Verification items for the finished model (mm, model axes). A direction names the side the tool comes from. Round coordinates to 2 decimals unless told otherwise and drop trailing zeros. Write each loop counter-clockwise with the first axis right and the second up, starting at its lowest first coordinate (ties: lowest second). Pieces come first, ordered by that corner, then holes. Notation, with made-up numbers: M -26,13 L 10,13 A18 cw 10,44 Z; hole C -18,57 d3. An arc over 180 degrees is marked long. One line per question, with ' | ' between items. Start each with the question number.
Q1. Gauge pin test, flat ends, axial feed: pin 1 (1.5 mm diameter, centred on x = -3.5, y = 11.5, fed in from -Z); pin 2 (3.5 mm diameter, centred on x = 14, y = -61.5, fed in from +Z). Record the tip position at first contact, or that the pin passes through.
Q2. Cross-section at C-C (z = 12.5). State how many separate pieces and enclosed holes the cut face has, then the cut area to 3 significant figures.
Q3. Tool access check on faces 1 (the face through (14, -61, 10)), 2 (the face through (25, -1, 7)). Record the directions out of +Z, -Z, +X, -X, +Y, -Y that give a thin tool (end or side, any length) a straight path to the whole face; none if there is none.
Q4. Cross-section at D-D (y = 21.18). Record the boundary of the cut face in (x, z).
Q5. Thickness scan on line 1 along Y through (x, z) = (-16.5, 12.85); line 2 along Y through (x, z) = (-10, 5.25); line 3 along X through (y, z) = (-14, 7.5). Record the ranges inside material, lowest first. Write a range as from..to.
Q6. Cross-section at B-B (y = 59.5). Record the boundary of the cut face in (x, z).
Q7. Release check for a two-part mould opening along Y. For faces 3 (the face through (15.784, -54.047, 12.535)), 4 (the face through (23, 67, 8)), 5 (the face through (0, -68, 7)) record: released by +Y, released by -Y, zero draft, split by the parting line, or undercut.
Q8. Cross-section at A-A (x = 16.5). Record the boundary of the cut face in (y, z).
from build123d import *

# Parameters (mm, degrees)
SKETCH_W        = 50
SKETCH_H        = 136
PAD_DEPTH       = 15
SKETCH001_R     = 2.75
POCKET_DEPTH    = 15.001
SKETCH002_R     = 5.5
POCKET001_DEPTH = 5
SKETCH003_R     = 2
POCKET002_DEPTH = 15.001
FILLET_R        = 5


with BuildPart() as part:
    # Sketch → Pad (new body)
    with BuildSketch(Plane.XY):
        Rectangle(SKETCH_W, SKETCH_H)
    extrude(amount=PAD_DEPTH)

    # Sketch001 (on Face6 of Pad) → Pocket (cut, through all)
    with BuildSketch(Plane.XY.offset(15)):
        with Locations((-16.5, 59.5)):
            Circle(SKETCH001_R)
        with Locations((16.5, 59.5)):
            Circle(SKETCH001_R)
        with Locations((16.5, -59.5)):
            Circle(SKETCH001_R)
        with Locations((-16.5, -59.5)):
            Circle(SKETCH001_R)
    extrude(amount=-POCKET_DEPTH, mode=Mode.SUBTRACT)

    # Sketch002 (on Face5 of Pocket) → Pocket001 (cut)
    with BuildSketch(Plane.XY.offset(15)):
        with Locations((-16.5, -59.5)):
            Circle(SKETCH002_R)
        with Locations((16.5, -59.5)):
            Circle(SKETCH002_R)
        with Locations((16.5, 59.5)):
            Circle(SKETCH002_R)
        with Locations((-16.5, 59.5)):
            Circle(SKETCH002_R)
    extrude(amount=-POCKET001_DEPTH, mode=Mode.SUBTRACT)

    # Sketch003 (on Face5 of Pocket001) → Pocket002 (cut, through all)
    with BuildSketch(Plane.XY.offset(15)):
        with Locations((10, 21.18)):
            Circle(SKETCH003_R)
        with Locations((-10, 21.18)):
            Circle(SKETCH003_R)
        with Locations((10, -14.82)):
            Circle(SKETCH003_R)
        with Locations((-10, -14.82)):
            Circle(SKETCH003_R)
    extrude(amount=-POCKET002_DEPTH, mode=Mode.SUBTRACT)

    # Fillet
    fillet_edges = [part.edges().sort_by_distance(p)[0] for p in [
        (-25, -68, 7.5),
        (-25, 68, 7.5),
        (25, 68, 7.5),
        (25, -68, 7.5),
    ]]
    fillet(fillet_edges, radius=FILLET_R)


solid = part.part
Determined:
1) pin 1: stops at z = 0 | pin 2: stops at z = 10
2) separate pieces: 1 | enclosed holes: 8 | area: 6,350 mm²
3) face 1: +Z | face 2: +Z, -Z, +X, +Y, -Y
4) outline: M -25,0 L -12,0 L -12,15 L -25,15 Z; M -8,0 L 8,0 L 8,15 L -8,15 Z; M 12,0 L 25,0 L 25,15 L 12,15 Z
5) line 1: y = -68..-65, -54..54, 65..68 | line 2: y = -68..-16.82, -12.82..19.18, 23.18..68 | line 3: x = -25..-11.82, -8.18..8.18, 11.82..25
6) outline: M -25,0 L -19.25,0 L -19.25,10 L -22,10 L -22,15 L -25,15 Z; M -13.75,0 L 13.75,0 L 13.75,10 L 11,10 L 11,15 L -11,15 L -11,10 L -13.75,10 Z; M 19.25,0 L 25,0 L 25,15 L 22,15 L 22,10 L 19.25,10 Z
7) face 3: undercut | face 4: released by +Y | face 5: released by -Y
8) outline: M -68,0 L -62.25,0 L -62.25,10 L -65,10 L -65,15 L -68,15 Z; M -56.75,0 L 56.75,0 L 56.75,10 L 54,10 L 54,15 L -54,15 L -54,10 L -56.75,10 Z; M 62.25,0 L 68,0 L 68,15 L 65,15 L 65,10 L 62.25,10 Z
